Autodesk Inventor part; units mm, degrees
ref_plane "YZ Plane" through (0, 0, 0) normal (1, 0, 0) x (0, 1, 0)
ref_plane "XZ Plane" through (0, 0, 0) normal (0, 1, 0) x (-1, 0, 0)
ref_plane "XY Plane" through (0, 0, 0) normal (0, 0, 1) x (1, 0, 0)
sketch "スケッチ1" plane through (0, 0, 0) normal (0, 0, 1) x (1, 0, 0)
  circle A0 centre (0, 0) radius 4
  dimension "d0" = 8
extrude "押し出し1" add sketch "スケッチ1" along normal blind 99.6
sketch "スケッチ2" plane through (0, 0, 99.6) normal (0, 0, 1) x (1, 0, 0)
  circle A0 centre (0, 0) radius 4
hole "穴1" at (0, 0, 99.6) direction (0, 0, -1) diameter 2.5 depth 12 tip angle 118
sketch "スケッチ3" plane through (0, 0, 0) normal (0, 0, -1) x (-1, 0, 0)
  circle A0 centre (0, 0) radius 4
hole "穴2" at (0, 0, 0) direction (0, 0, 1) diameter 2.5 depth 12 tip angle 118
properties part number "シャフト" material "ポリカーボネート、クリア"
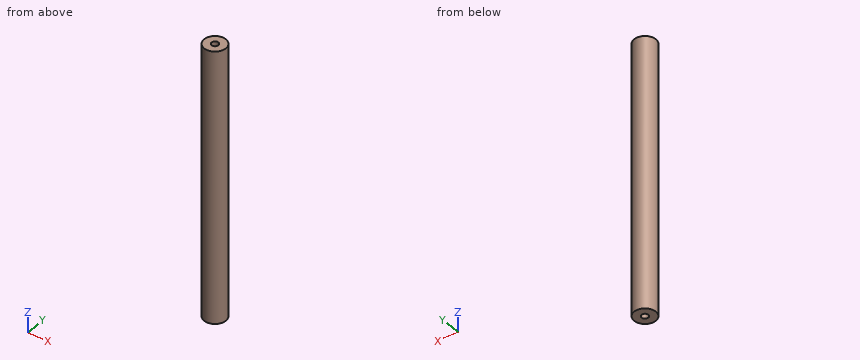
Geometry check sheet. Reference: the model listing, model coordinates, mm. Coordinates: 2 decimals unless noted, no trailing zeros. Order: outer loops, then holes, each group sorted by start corner. A loop starts at its lowest first (then second) coordinate and runs counter-clockwise, first axis right, second up. Notation, with made-up numbers: M -22.5,51 L 23.5,51 A25 cw 23.5,66 Z; hole C 70,-28 d4. An arc over 180 degrees is marked long. Use CSV: the item, a comma, the result in double quotes.
Item 1: Gauge pin test, flat end, axial feed: pin 1 Ø1.5 at (x, y) = (0, 0) entering from +Z. Record the tip position at first contact, or that the pin passes through.
Returned:
pin 1,"stops at z = 87.3"
Item 2: Cross-section at C-C on z = 67. Record the cut outline in (x, y), then the cut area to 3 significant figures.
Returned:
outline,"C 0,0 d8"
area,"50.3 mm2"
Item 3: Thickness scan on line 1 along Y through (x, z) = (0, 9.5); line 2 along Y through (x, z) = (-0.25, 81); line 3 along Y through (x, z) = (3.5, 72.5). Record the ranges inside material, lowest first.
Returned:
line 1,"y = -4 to -1.25, 1.25 to 4"
line 2,"y = -3.99 to 3.99"
line 3,"y = -1.94 to 1.94"
Item 4: Cross-section at B-B on y = 3. Record the cut outline in (x, z).
Returned:
outline,"M -2.65,0 L 2.65,0 L 2.65,99.6 L -2.65,99.6 Z"
Item 5: Cross-section at A-A on x = 2.25. Record the cut outline in (y, z).
Returned:
outline,"M -3.31,0 L 3.31,0 L 3.31,99.6 L -3.31,99.6 Z"
